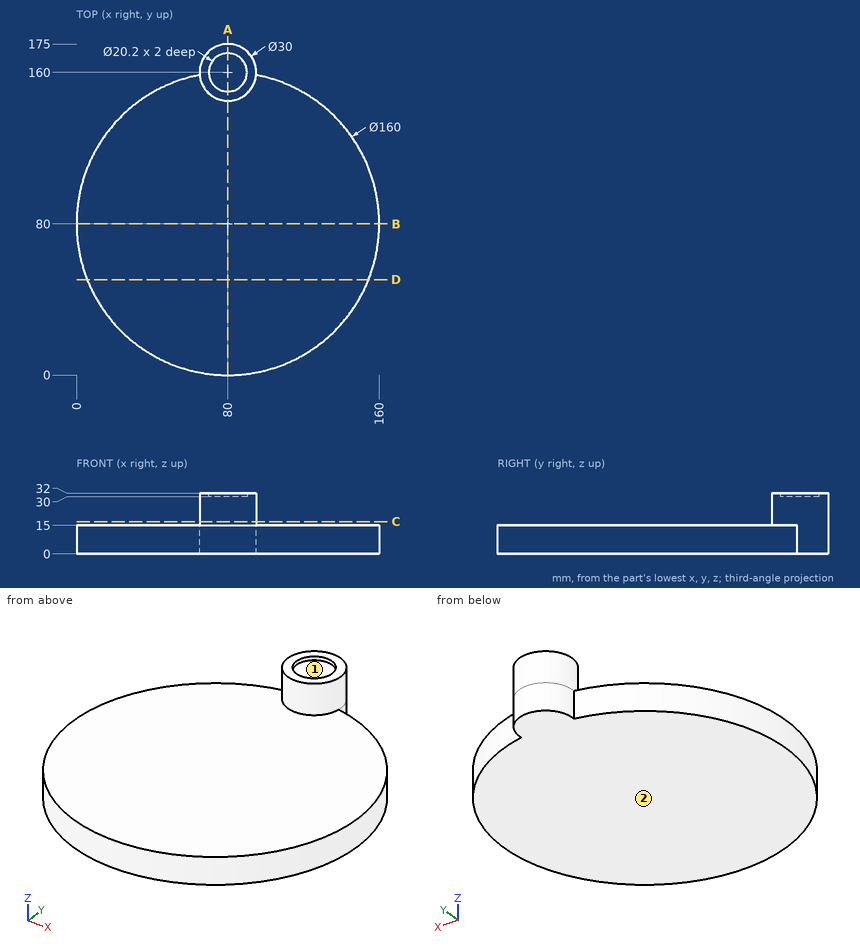
Job drawing, mm, ordinate dimensions from the low corner. One solid piece. Give positions to 0.01 mm unless a question says otherwise; leave off trailing zeros. Loops run counter-clockwise (first coordinate to the right, second up) from the corner with the lowest first, then second, coordinate; pieces in that order, holes last. Notation, with made-up numbers: (-32.75, 42.5) -> (13.25, 42.5) arc R23 ccw to (13.25, 65.5) -> close; hole circle Ø10 at (62, 61.5). An arc over 180 degrees is marked (long way). Use a Markdown table: item, result. Add a question column.
(1) Mould opens along Y. For the marked faces 1 and 2 say: +Y half, -Y half, draft (parallel to the pull), parting line (faces both ways), or undercut.
(2) Slice it at B-B on y = 80. List the corners of the cut face in (x, z), and give its area (3 significant figures).
(3) Drop flat-ended pins along their axis: pin 1 Ø16 at (x, y) = (80, 160) entering from +Z; pin 2 Ø4 at (x, z) = (94, 14.5) entering from -Y; pin 3 Ø2 at (y, z) = (136, 11.5) entering from +X. Give the stop position or say it passes through.
(4) Wall check: line 1 along Y through (x, z) = (80, 31.6); line 2 along Z through (x, y) = (94.5, 23); line 3 along X through (y, z) = (65.5, 12.5). Give the ranges that are in metal, low to high.
(5) Slice it at D-D on y = 50.5. List the corners of the cut face in (x, z).
(6) Slice it at C-C on z = 17. List the corners of the cut face in (x, y).
(7) Slice it at A-A on x = 80. List the corners of the cut face in (y, z), and give its area (3 significant figures).
Filled sheet:
| question | item | result |
|---|---|---|
| 1 | face 1 | undercut |
| 1 | face 2 | draft |
| 2 | outline | (0, 0) -> (160, 0) -> (160, 15) -> (0, 15) -> close |
| 2 | area | 2,400 mm2 |
| 3 | pin 1 | z = 30 |
| 3 | pin 2 | y = 0.91 |
| 3 | pin 3 | x = 138.09 |
| 4 | line 1 | 145 to 149.9, 170.1 to 175 |
| 4 | line 2 | 0 to 15 |
| 4 | line 3 | 1.33 to 158.67 |
| 5 | outline | (5.64, 0) -> (154.36, 0) -> (154.36, 15) -> (5.64, 15) -> close |
| 6 | outline | circle Ø30 at (80, 160) |
| 7 | outline | (0, 0) -> (175, 0) -> (175, 32) -> (170.1, 32) -> (170.1, 30) -> (149.9, 30) -> (149.9, 32) -> (145, 32) -> (145, 15) -> (0, 15) -> close |
| 7 | area | 3,090 mm2 |
